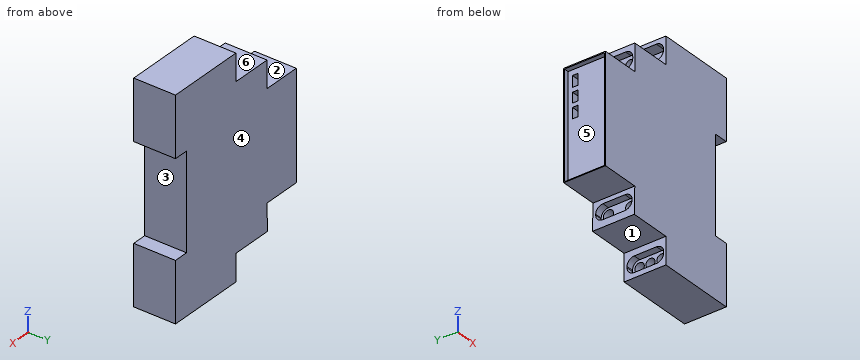
```python
from build123d import *

# Parameters (mm, degrees)
F1_DEPTH  = 17.5
F4_DEPTH  = 5
F6_DEPTH  = 3
F8_DEPTH  = 3
F9_W      = 16.8058317795
F9_H      = 44.2914962769
F10_DEPTH = 2
F2_R      = 2.117891982
F2_R_2    = 2.2502095604
F2_R_3    = 2.1412189154
F2_R_4    = 1.9250274961
F2_R_5    = 1.9886102938
F2_R_6    = 1.8999785502
F2_R_7    = 1.9125474789
F11_DEPTH = 45
F13_DEPTH = 3
F14_W     = 2.2663704585
F14_H     = 4.6991482377
F14_H_2   = 4.3204948306
F14_H_3   = 4.5327991247
F15_DEPTH = 3


with BuildPart() as f1:
    # F0 (on Front) → F1 (new body)
    with BuildSketch(Plane.XZ):
        Polygon((-29.036315158, 123.5913918912), (-62.036315158, 123.5913918912), (-62.036315158, 112.3413918912), (-79.036315158, 112.3413918912), (-79.036315158, 101.0913918912), (-95.036315158, 101.0913918912), (-95.036315158, 56.0913918912), (-79.036315158, 56.0913918912), (-79.3131489307, 44.8413918912), (-62.036315158, 44.8413918912), (-62.036315158, 33.5913918912), (-29.036315158, 33.5913918912), (-29.036315158, 58.5913918912), (-35.036315158, 58.5913918912), (-35.036315158, 98.5913918912), (-29.036315158, 98.5913918912), align=None)
    extrude(amount=F1_DEPTH)

    # F3 (on face) → F4 (cut)
    with BuildSketch(Plane(origin=(-62.036315158, 0, 0), x_dir=(0, -1, 0), z_dir=(-1, 0, 0))):
        with BuildLine():
            Line((13.4917167276, 121.9224523306), (4.209778944, 121.9224523306))
            ThreePointArc((4.209778944, 121.9224523306), (2.0884586005, 121.0437726741), (1.209778944, 118.9224523306))
            Line((1.209778944, 118.9224523306), (1.209778944, 118.5100823641))
            ThreePointArc((1.209778944, 118.5100823641), (2.0884586005, 116.3887620205), (4.209778944, 115.5100823641))
            Line((4.209778944, 115.5100823641), (13.4917167276, 115.5100823641))
            ThreePointArc((13.4917167276, 115.5100823641), (15.6130370712, 116.3887620205), (16.4917167276, 118.5100823641))
            Line((16.4917167276, 118.5100823641), (16.4917167276, 118.9224523306))
            ThreePointArc((16.4917167276, 118.9224523306), (15.6130370712, 121.0437726741), (13.4917167276, 121.9224523306))
        make_face()
    extrude(amount=-F4_DEPTH, mode=Mode.SUBTRACT)

    # F5 (on face) → F6 (cut)
    with BuildSketch(Plane(origin=(-79.036315158, 0, 0), x_dir=(0, -1, 0), z_dir=(-1, 0, 0))):
        with BuildLine():
            Line((13.656557098, 110.2756986618), (3.9331587353, 110.2756986618))
            ThreePointArc((3.9331587353, 110.2756986618), (1.8118383917, 109.3970190054), (0.9331587353, 107.2756986618))
            Line((0.9331587353, 107.2756986618), (0.9331587353, 106.5890877247))
            ThreePointArc((0.9331587353, 106.5890877247), (1.8118383917, 104.4677673811), (3.9331587353, 103.5890877247))
            Line((3.9331587353, 103.5890877247), (13.656557098, 103.5890877247))
            ThreePointArc((13.656557098, 103.5890877247), (15.7778774416, 104.4677673811), (16.656557098, 106.5890877247))
            Line((16.656557098, 106.5890877247), (16.656557098, 107.2756986618))
            ThreePointArc((16.656557098, 107.2756986618), (15.7778774416, 109.3970190054), (13.656557098, 110.2756986618))
        make_face()
    extrude(amount=-F6_DEPTH, mode=Mode.SUBTRACT)

    # F7 (on face) → F8 (cut)
    with BuildSketch(Plane(origin=(-62.036315158, 0, 0), x_dir=(0, -1, 0), z_dir=(-1, 0, 0))):
        with BuildLine():
            ThreePointArc((1.2264838442, 38.6837883592), (2.1051635007, 36.5624680156), (4.2264838442, 35.6837883592))
            Line((4.2264838442, 35.6837883592), (13.5701508522, 35.6837883592))
            ThreePointArc((13.5701508522, 35.6837883592), (15.6914711958, 36.5624680156), (16.5701508522, 38.6837883592))
            Line((16.5701508522, 38.6837883592), (16.5701508522, 39.2147824168))
            ThreePointArc((16.5701508522, 39.2147824168), (15.6914711958, 41.3361027604), (13.5701508522, 42.2147824168))
            Line((13.5701508522, 42.2147824168), (4.2264838442, 42.2147824168))
            ThreePointArc((4.2264838442, 42.2147824168), (2.1051635007, 41.3361027604), (1.2264838442, 39.2147824168))
            Line((1.2264838442, 39.2147824168), (1.2264838442, 38.6837883592))
        make_face()
    extrude(amount=-F8_DEPTH, mode=Mode.SUBTRACT)

    # F9 (on face) → F10 (cut)
    with BuildSketch(Plane(origin=(-95.036315158, 0, 0), x_dir=(0, -1, 0), z_dir=(-1, 0, 0))):
        with Locations((8.6868142389, 78.5176903009)):
            Rectangle(F9_W, F9_H)
    extrude(amount=-F10_DEPTH, mode=Mode.SUBTRACT)

    # F2 (on face) → F11 (cut)
    with BuildSketch(Plane(origin=(-95.036315158, 0, 0), x_dir=(0, -1, 0), z_dir=(-1, 0, 0))):
        with Locations((4.1773817502, 118.7390312552)):
            Circle(F2_R)
        with Locations((13.2942087948, 118.7390312552)):
            Circle(F2_R_2)
        with Locations((4.1773817502, 106.985270977)):
            Circle(F2_R_3)
        with Locations((13.2942087948, 106.985270977)):
            Circle(F2_R_4)
        with Locations((4.2668927927, 51.1149987578)):
            Circle(F2_R_3)
        with Locations((13.3837198373, 51.1149987578)):
            Circle(F2_R_4)
        with Locations((4.1773817502, 39.1167402267)):
            Circle(F2_R_5)
        with Locations((8.744363673, 39.1167402267)):
            Circle(F2_R_6)
        with Locations((13.2942087948, 39.1167402267)):
            Circle(F2_R_7)
    extrude(amount=-F11_DEPTH, mode=Mode.SUBTRACT)

    # F12 (on face) → F13 (cut)
    with BuildSketch(Plane(origin=(-80.3679161841, 0, 1.9776491945), x_dir=(0, -1, 0), z_dir=(-0.9996973742, 0, 0.0245999996))):
        with BuildLine():
            ThreePointArc((16.4354741573, 49.2703006864), (15.5567945009, 51.3916210299), (13.4354741573, 52.2703006864))
            Line((13.4354741573, 52.2703006864), (4.2163297506, 52.2703006864))
            ThreePointArc((4.2163297506, 52.2703006864), (2.095009407, 51.3916210299), (1.2163297506, 49.2703006864))
            Line((1.2163297506, 49.2703006864), (1.2163297506, 48.8921268582))
            ThreePointArc((1.2163297506, 48.8921268582), (2.095009407, 46.7708065147), (4.2163297506, 45.8921268582))
            Line((4.2163297506, 45.8921268582), (13.4354741573, 45.8921268582))
            ThreePointArc((13.4354741573, 45.8921268582), (15.5567945009, 46.7708065147), (16.4354741573, 48.8921268582))
            Line((16.4354741573, 48.8921268582), (16.4354741573, 49.2703006864))
        make_face()
    extrude(amount=-F13_DEPTH, mode=Mode.SUBTRACT)

    # F14 (on face) → F15 (cut)
    with BuildSketch(Plane(origin=(-93.036315158, 0, 0), x_dir=(0, -1, 0), z_dir=(-1, 0, 0))):
        with Locations((3.2347693341, 96.0811041296)):
            Rectangle(F14_W, F14_H)
        with Locations((3.2347693341, 89.7187851369)):
            Rectangle(F14_W, F14_H_2)
        with Locations((3.2347693341, 83.6331695318)):
            Rectangle(F14_W, F14_H_3)
    extrude(amount=-F15_DEPTH, mode=Mode.SUBTRACT)


solid = f1.part
```
Here's how the part is built. I have some questions about the finished solid (model axes, mm). Face numbers are marked on the shaded views. A direction names the side the tool comes from. Give positions to 0.01 mm unless a question says otherwise; leave off trailing zeros. Loops run counter-clockwise (first coordinate to the right, second up) from the corner with the lowest first, then second, coordinate; pieces in that order, holes last. Notation, with made-up numbers: M -5.75,80.25 L 6.25,80.25 A18 ccw 6.25,97.25 Z; hole C 65.5,6 d10. An arc over 180 degrees is marked long. Use one line per item in the form item = value. Start each with the question number.
Q1. Thinking about a two-plate mould opening in Y: for the marked faces 4, 5 and 6, which applies, +Y half, -Y half, draft (parallel to the pull), parting line (faces both ways), or undercut?
Q2. If we section it at B-B (x = -53): State how many separate pieces and enclosed holes the cut face has, then the cut area to 3 significant figures.
Q3. Will these pins go through, and if not, where does the flat tip stop? pin 1 Ø5 at (x, y) = (-80.5, -14) entering from -Z; pin 2 Ø3.5 at (y, z) = (-3.5, 107) entering from -X; pin 3 Ø5.5 at (y, z) = (-8, 105.5) entering from -X.
Q4. If we section it at C-C (x = -80.5): Write out the boundary of the cut face in (y, z), then the cut area to 4 significant figures.
Q5. Which directions (+Z, -Z, +X, -X, +Y, -Y) give clear straight access to the entire face, cutting with the end or side of a thin tool? Please do the marked faces 1, 2 and 3.
Q6. I need wall thicknesses on line 1 along Z through (x, y) = (-61, -10.75); line 2 along Z through (x, y) = (-86, -14.25); line 3 along X through (y, z) = (-15.5, 54.5). Which ranges of each line are inside material? Lowest first, please.
Q7. If we section it at D-D (z = 63): Write out the boundary of the cut face in (x, y).
Q8. If we section it at A-A (z = 97): Write out the boundary of the cut face in (x, y).
Taken from the geometry:
q1.face_4 = +Y half
q1.face_5 = undercut
q1.face_6 = draft
q2.separate_pieces = 1
q2.enclosed_holes = 9
q2.area = 1,460 mm^2
q3.pin_1 = 44.84
q3.pin_2 = -76.04
q3.pin_3 = -79.04
q4.outline = M -17.5,56.09 L 0,56.09 L 0,101.09 L -17.5,101.09 Z
q4.area = 787.5 mm^2
q5.face_1 = -Z, -X, +Y, -Y
q5.face_2 = +Z, -X, +Y, -Y
q5.face_3 = +X, +Y, -Y
q6.line_1 = 33.59 to 35.68, 42.21 to 115.51, 121.92 to 123.59
q6.line_2 = 56.09 to 101.09
q6.line_3 = -79.08 to -29.04
q7.outline = M -95.04,-17.5 L -35.04,-17.5 L -35.04,0 L -95.04,0 L -95.04,-0.28 L -93.04,-0.28 L -93.04,-17.09 L -95.04,-17.09 Z
q8.outline = M -95.04,-17.5 L -35.04,-17.5 L -35.04,0 L -95.04,0 L -95.04,-0.28 L -93.04,-0.28 L -93.04,-2.1 L -90.04,-2.1 L -90.04,-4.37 L -93.04,-4.37 L -93.04,-17.09 L -95.04,-17.09 Z
